Verification items for the finished model (mm, model axes). A direction names the side the tool comes from. Round coordinates to 2 decimals unless told otherwise and drop trailing zeros. Write each loop counter-clockwise with the first axis right and the second up, starting at its lowest first coordinate (ties: lowest second). Pieces come first, ordered by that corner, then holes. Notation, with made-up numbers: (27, 13.25) -> (40, 13.25) arc R19 ccw to (40, 48.25) -> close; hole circle Ø1 at (-3, -22.75). An arc over 180 degrees is marked (long way). Use CSV: the item, a comma, the result in double quotes.
```python
from build123d import *

# Parameters (mm, degrees)
ESQUISSE1_R             = 190
BOSS_EXTRU_1_DEPTH      = 5
ENL_V_MAT_EXTRU_1_DEPTH = 5
ENL_V_MAT_EXTRU_2_DEPTH = 10


with BuildPart() as part:
    # Esquisse1 → Boss.-Extru.1 (new body)
    with BuildSketch(Plane.XY):
        Circle(ESQUISSE1_R)
    extrude(amount=-BOSS_EXTRU_1_DEPTH)

    # Esquisse2 → Enlèv. mat.-Extru.1 (cut)
    with BuildSketch(Plane.XY):
        Polygon((-15, 150), (-15, 90), (15, 90), (15, 150), (30, 150), (30, 180), (-30, 180), (-30, 150), align=None)
        Polygon((30, -180), (30, -150), (15, -150), (15, -90), (-15, -90), (-15, -150), (-30, -150), (-30, -180), align=None)
        Polygon((180, 30), (150, 30), (150, 15), (90, 15), (90, -15), (150, -15), (150, -30), (180, -30), align=None)
        Polygon((-180, -30), (-150, -30), (-150, -15), (-90, -15), (-90, 15), (-150, 15), (-150, 30), (-180, 30), align=None)
    extrude(amount=-ENL_V_MAT_EXTRU_1_DEPTH, mode=Mode.SUBTRACT)

    # Esquisse3 → Enlèv. mat.-Extru.2 (cut)
    with BuildSketch(Plane.XY):
        Polygon((-88.741430887, 49.850557922), (-49.850557922, 88.741430887), (-113.490168229, 152.381041194), (-120.561236041, 159.452109006), (-159.452109006, 120.561236041), (-152.381041194, 113.490168229), align=None)
    extrude(amount=-ENL_V_MAT_EXTRU_2_DEPTH, mode=Mode.SUBTRACT)


solid = part.part
```
Q1. Access from +Z, -Z, +X, -X, +Y, -Y to the whole of each face (thin tool, end or side, straight path). Record for faces 1 (the flat face through (-69.57, 69.02, -2.46)), 2 (the flat face through (-3, 3, -5)).
Filled in:
face 1,"+Z, -Z"
face 2,"-Z, +X, -X, +Y, -Y"
Q2. Section check D-D (x = 108). Record the cut outline in (y, z), plus the area to 3 significant figures.
Filled in:
outline,"(-156.32, -5) -> (-15, -5) -> (-15, 0) -> (-156.32, 0) -> close; (15, -5) -> (156.32, -5) -> (156.32, 0) -> (15, 0) -> close"
area,"1,410 mm²"
Q3. Material ranges on L1, parallel to X at y = 95, z = -4.2; L2, parallel to X at y = -7, z = -2.95; L3, parallel to Y at x = 14.5, z = -3.1, recorded low to high.
Filled in:
L1,"-164.54 to -133.89, -56.11 to -15, 15 to 164.54"
L2,"-189.87 to -180, -90 to 90, 180 to 189.87"
L3,"-189.45 to -180, -90 to 90, 180 to 189.45"
Q4. Go/stop test with flat-tipped pins: P1, Ø1, axis at y = 149.5, z = -3.5, coming from the +X side; P2, Ø2.5, axis at y = 22, z = -2.5, coming from the +X side; P3, Ø1.5, axis at x = 136, z = -3.5, coming from the +Y side. Record where each tip stops, or that it passes through.
Filled in:
P1,"x = 117.89"
P2,"x = 188.86"
P3,"y = 133.44"
Q5. Section check A-A (y = 0). Record the cut outline in (x, z).
Filled in:
outline,"(-190, -5) -> (-180, -5) -> (-180, 0) -> (-190, 0) -> close; (-90, -5) -> (90, -5) -> (90, 0) -> (-90, 0) -> close; (180, -5) -> (190, -5) -> (190, 0) -> (180, 0) -> close"
Q6. Section check C-C (y = -162). Record the cut outline in (x, z).
Filled in:
outline,"(-99.28, -5) -> (-30, -5) -> (-30, 0) -> (-99.28, 0) -> close; (30, -5) -> (99.28, -5) -> (99.28, 0) -> (30, 0) -> close"
